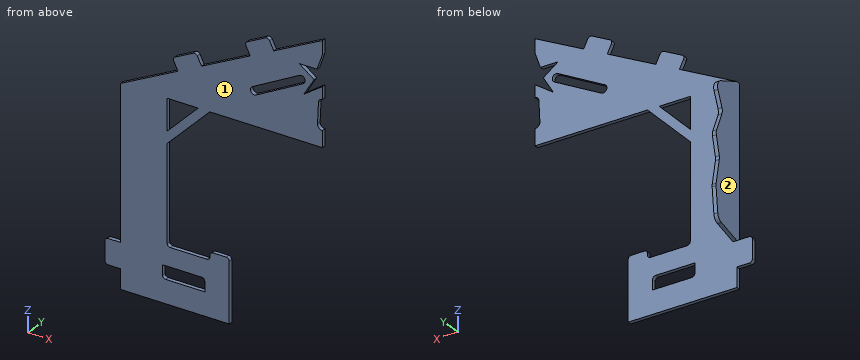
```python
from build123d import *

# Parameters (mm, degrees)
F1_DEPTH  = 3.175
F2_W      = 15.748
F2_H      = 6.35
F2_W_2    = 12.7
F2_H_2    = 20.32
F3_DEPTH  = 3.175
F4_R      = 2.54
F5_W      = 34.5431789756
F5_H      = 10.5385929346
F6_DEPTH  = 3.176
F8_DEPTH  = 3.175
F9_R      = 6.35
F10_R     = 2.54
F12_W     = 206.8448513746
F12_H     = 268.8337340951
F13_DEPTH = 28.5116125674


with BuildPart() as f1:
    # F0 (on Front) → F1 (new body)
    with BuildSketch(Plane.XZ):
        Polygon((0, 82.55), (0, 0), (127, 0), (127, -114.3), (76.2, -114.3), (76.2, -158.75), (165.1, -158.75), (165.1, 0), align=None)
    extrude(amount=-F1_DEPTH)

    # F2 (on face) → F3 (join, through all)
    with BuildSketch(Plane.XZ):
        Polygon((44.3009787702, 71.7587359406), (39.7572886399, 62.67135568), (59.0679716936, 53.0160141532), (63.6116618239, 62.1033944137), align=None)
        Polygon((122.6796335175, 32.5694085669), (103.3689504639, 42.2247500938), (98.8252603336, 33.1373698332), (118.1359433873, 23.4820283064), align=None)
        with Locations((84.074, -111.125)):
            Rectangle(F2_W, F2_H)
        with Locations((171.45, -132.715)):
            Rectangle(F2_W_2, F2_H_2)
        Polygon((127, -25.4), (101.6, 0), (92.075, 0), (127, -34.925), align=None)
    extrude(amount=-F3_DEPTH)

    # F4
    f4_edges = [f1.edges().sort_by_distance(p)[0] for p in [
        (177.8, 1.5875, -142.875),
        (177.8, 1.5875, -122.555),
        (91.948, 1.5875, -107.95),
        (122.679634, 1.5875, 32.569409),
        (63.611662, 1.5875, 62.103394),
        (103.36895, 1.5875, 42.22475),
        (44.300979, 1.5875, 71.758736),
        (76.2, 1.5875, -107.95),
        (91.948, 1.5875, -114.3),
        (127, 1.5875, -114.3),
    ]]
    fillet(f4_edges, radius=F4_R)

    # F5 (on face) → F6 (cut, through all)
    with BuildSketch(Plane.XZ):
        Polygon((4.4021862559, 59.1385737062), (0, 71.4375), (0, 47.0566861331), (15.08702501, 36.7185198719), (6.7811906338, 50.3608770669), (18.8778863964, 59.1385737062), align=None)
        with BuildLine():
            Line((15.7880578146, 44.4895698524), (54.4423557636, 24.1893212834))
            ThreePointArc((54.4423557636, 24.1893212834), (58.4390000122, 25.6523165849), (57.3894998938, 29.7768856537))
            Line((57.3894998938, 29.7768856537), (18.7659755805, 50.0979274743))
            ThreePointArc((18.7659755805, 50.0979274743), (14.4600820897, 48.7894806012), (15.7880578146, 44.4895698524))
        make_face()
        with BuildLine():
            Line((3.9643459731, 17.3010716776), (3.1714767785, 34.1172288808))
            ThreePointArc((3.1714767785, 34.1172288808), (2.1915586368, 36.2650197343), (0, 37.1426961303))
            Line((0, 37.1426961303), (0, 13.1454057395))
            ThreePointArc((0, 13.1454057395), (2.871654505, 14.3747074435), (3.9643459731, 17.3010716776))
        make_face()
        with Locations((113.4665496647, -134.7029581666)):
            Rectangle(F5_W, F5_H)
    extrude(amount=-F6_DEPTH, mode=Mode.SUBTRACT)

    # F7 (on face) → F8 (join)
    with BuildSketch(Plane.YZ.offset(165.1)):
        Polygon((28.5750000001, -10.4543957859), (3.175, 0), (3.1750000001, -122.555), (25.9204413742, -115.6956553459), (28.5750000001, -90.5212983489), (24.2223335625, -68.0457651615), (28.5750000001, -50.012152642), (20.3100345423, -30.5349558611), align=None)
    extrude(amount=-F8_DEPTH)

    # F9
    f9_edges = [f1.edges().sort_by_distance(p)[0] for p in [
        (163.5125, 28.575, -10.454396),
        (163.5125, 20.310035, -30.534956),
        (163.5125, 28.575, -50.012153),
        (163.5125, 24.222334, -68.045765),
        (163.5125, 28.575, -90.521298),
        (163.5125, 25.920441, -115.695655),
    ]]
    fillet(f9_edges, radius=F9_R)

    # F10
    f10_edges = [f1.edges().sort_by_distance(p)[0] for p in [
        (96.19496, 1.5875, -129.433662),
        (130.738139, 1.5875, -139.972255),
    ]]
    fillet(f10_edges, radius=F10_R)

    # F11: F1 across plane


with BuildPart() as f1_1:
    add(f1.part)
    add(f1.part.mirror(Plane.YZ))

    # F12 (on Front) → F13 (cut, through all)
    with BuildSketch(Plane.XZ):
        with Locations((103.4224256873, -33.929746598)):
            Rectangle(F12_W, F12_H)
    extrude(amount=-F13_DEPTH, mode=Mode.SUBTRACT)


solid = f1_1.part
```
The listing builds one solid part. Answer for the finished solid, in the listing's coordinates (mm). Face numbers are marked on the shaded views. A direction names the side the tool comes from. Coordinates: 2 decimals unless noted, no trailing zeros. Write each loop counter-clockwise with the first axis right and the second up, starting at its lowest first coordinate (ties: lowest second). Pieces come first, ordered by that corner, then holes. Notation, with made-up numbers: (52, -38) -> (75, -38) arc R31 cw to (75, -2) -> close; hole circle Ø1 at (1.25, 40.25). An arc over 180 degrees is marked (long way). Write each question's results on one line, items separated by ' | '. Start each with the question number.
1) A cutting plane is placed at A-A (x = -139.5). Determine the outline of the cut face in (y, z) (3 decimals).
2) Flat-ended cylindrical pins translate along their axes: pin 1 Ø1.6 at (x, y) = (-171, 1.5) entering from -Z (3 decimals); pin 2 Ø4 at (x, y) = (-72, 3) entering from +Z; pin 3 Ø10 at (y, z) = (14.5, -61.5) entering from +X (3 decimals). Find the tip coordinate at first contact, or state that the pin passes through.
3) A tool of negligible diameter and unlimited length cuts with its end or side. For the marked faces 1 and 2, from which of +Z, -Z, +X, -X, +Y, -Y can it reach the whole face along a straight path? Write none if from no direction.
4) Straight lines are drawn through the part: probe 1 along X at (y, z) = (13.5, -83) (3 decimals); probe 2 along Y at (x, z) = (-104, 31) (3 decimals); probe 3 along Z at (x, y) = (-140, 1.5). For each, find the intervals that lie inside material, in ascending order.
5) A cutting plane is placed at B-B (z = 10.5). Determine the outline of the cut face in (x, y) (3 decimals).
6) A cutting plane is placed at C-C (z = -100.5). Determine the outline of the cut face in (x, y) (3 decimals).
Values follow:
1) outline: (0, -158.75) -> (3.175, -158.75) -> (3.175, 12.8) -> (0, 12.8) -> close
2) pin 1: z = -142.875 | pin 2: z = 47.55 | pin 3: x = -161.925
3) face 1: +Z, -Z, +X, -X, -Y | face 2: +Z, -X, +Y, -Y
4) probe 1: -165.1 to -161.925 | probe 2: 0 to 3.175 | probe 3: -158.75 to 12.55
5) outline: (-144.1, 0) -> (0, 0) -> (0, 3.175) -> (-144.1, 3.175) -> close
6) outline: (-165.1, 0) -> (-127, 0) -> (-127, 3.175) -> (-161.925, 3.175) -> (-161.925, 27.523) -> (-165.1, 27.523) -> close
